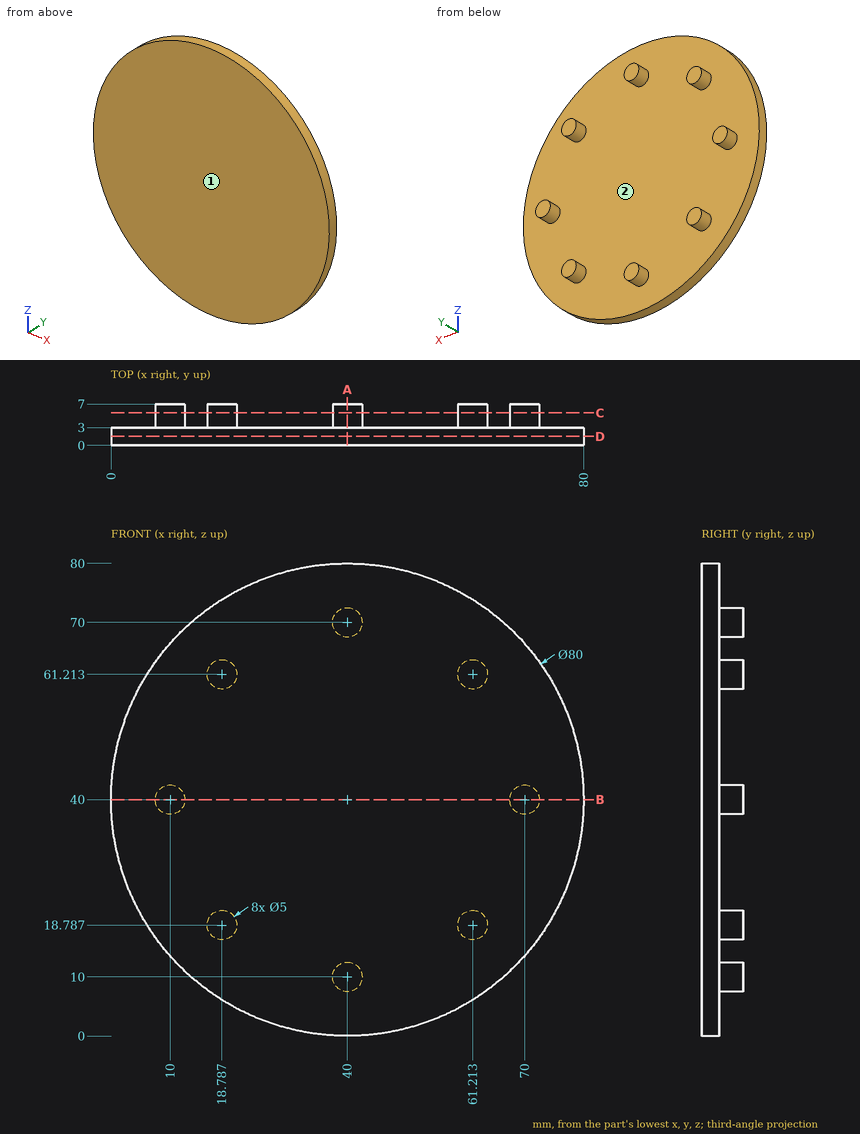
Verification items for this drawing (mm, ordinates from the low corner). A direction names the side the tool comes from. Round coordinates to 2 decimals unless told otherwise and drop trailing zeros. Write each loop counter-clockwise with the first axis right and the second up, starting at its lowest first coordinate (ties: lowest second). Pieces come first, ordered by that corner, then holes. Notation, with made-up numbers: (23.25, 89) - (69.25, 89) arc R31 cw to (69.25, 117) - close; hole circle Ø1 at (65, -9). An arc over 180 degrees is marked (long way). Answer as a JSON object with one key per item and string values. Group by question number.
Q1. Section check A-A, the plane x = 40. Enter the section's corners in (y, z), plus the area to 3 significant figures.
Q2. Go/stop test with flat-tipped pins: pin 1 Ø1 at (y, z) = (2.5, 56) entering from -X (1 decimal); pin 2 Ø3 at (x, y) = (71.5, 1) entering from +Z; pin 3 Ø1.5 at (x, z) = (51, 24) entering from +Y. Record where each tip stops, or that it passes through.
Q3. Section check D-D, the plane y = 1.5. Enter the section's corners in (x, z), plus the area to 3 significant figures.
Q4. Tool access check on the marked faces 1 and 2. Record the directions out of +Z, -Z, +X, -X, +Y, -Y that give a thin tool (end or side, any length) a straight path to the whole face; none if there is none.
Q5. Section check C-C, the plane y = 5.5. Enter the section's corners in (x, z), plus the area to 3 significant figures.
Q6. Section check B-B, the plane z = 40. Enter the section's corners in (x, y).
Q7. Thickness scan on line 1 (Y direction, x = 53, z = 33); line 2 (Z direction, x = 70, y = 3.5); line 3 (Z direction, x = 26.5, y = 0.5). Record the ranges inside material, lowest first.
Found:
{
 "1": {"outline": "(0, 0) - (3, 0) - (3, 7.5) - (7, 7.5) - (7, 12.5) - (3, 12.5) - (3, 67.5) - (7, 67.5) - (7, 72.5) - (3, 72.5) - (3, 80) - (0, 80) - close", "area": "280 mm^2"},
 "2": {"pin 1": "stops at x = 3.1", "pin 2": "stops at z = 66.46", "pin 3": "stops at y = 3"},
 "3": {"outline": "circle Ø80 at (40, 40)", "area": "5,030 mm^2"},
 "4": {"face 1": "+Z, -Z, +X, -X, -Y", "face 2": "+Y"},
 "5": {"outline": "circle Ø5 at (10, 40); circle Ø5 at (18.79, 18.79); circle Ø5 at (18.79, 61.21); circle Ø5 at (40, 10); circle Ø5 at (40, 70); circle Ø5 at (61.21, 18.79); circle Ø5 at (61.21, 61.21); circle Ø5 at (70, 40)", "area": "157 mm^2"},
 "6": {"outline": "(0, 0) - (80, 0) - (80, 3) - (72.5, 3) - (72.5, 7) - (67.5, 7) - (67.5, 3) - (12.5, 3) - (12.5, 7) - (7.5, 7) - (7.5, 3) - (0, 3) - close"},
 "7": {"line 1": "y = 0 to 3", "line 2": "z = 37.5 to 42.5", "line 3": "z = 2.35 to 77.65"}
}
